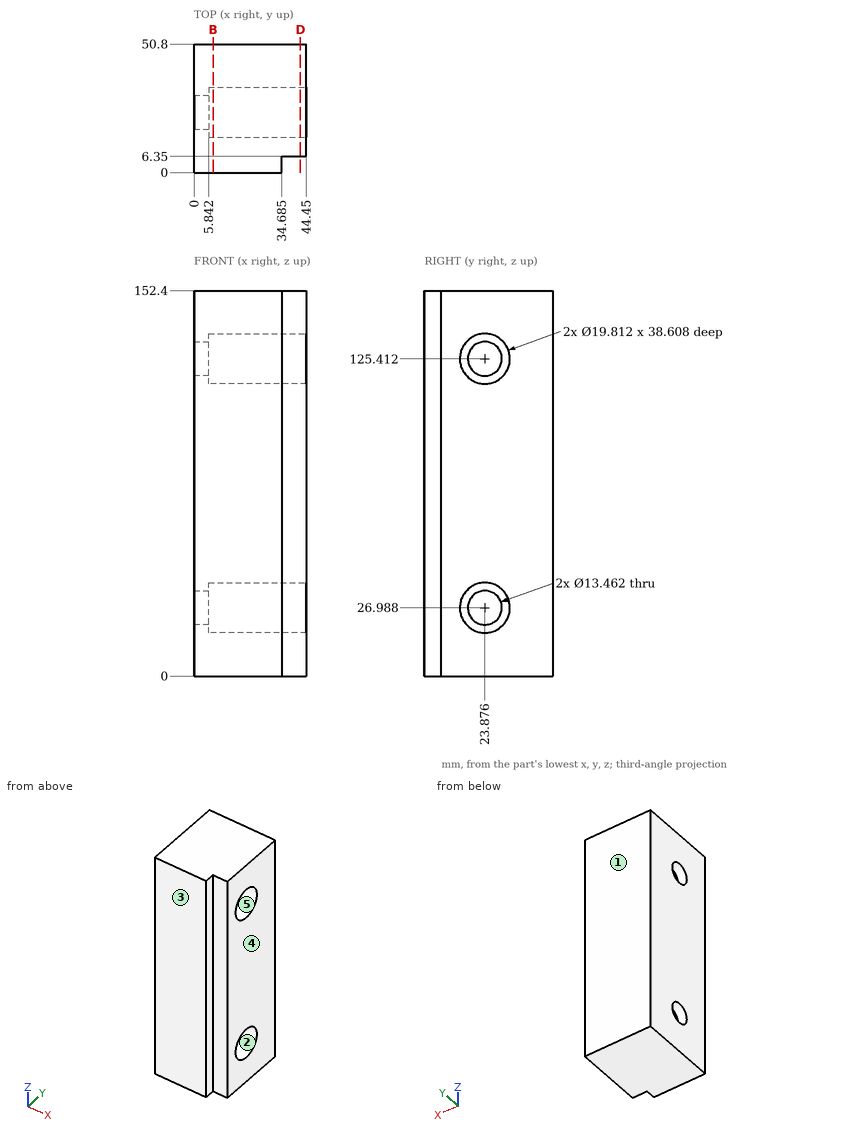
Drawing for the job (mm, zero at the part's lowest x, y, z). A direction names the side the tool comes from. Round coordinates to 2 decimals unless told otherwise and drop trailing zeros. Write each loop counter-clockwise with the first axis right and the second up, starting at its lowest first coordinate (ties: lowest second). Pieces come first, ordered by that corner, then holes. Notation, with made-up numbers: (50, 25) - (65, 25) arc R24 ccw to (65, 47) - close; hole circle Ø10 at (30, 16). An arc over 180 degrees is marked (long way). Return JSON: item names as keys, results as strings. Group by question number.
Item 1: Band-saw the part on D-D on x = 42. State how many separate pieces and enclosed holes the cut face has, plus the area to 3 significant figures.
Item 2: Flat gauge pins, fed straight in: pin 1 Ø8 at (x, z) = (40, 95.5) entering from -Y; pin 2 Ø16 at (y, z) = (24, 125) entering from +X. Where does each tip first touch, or does it go through?
Item 3: Mould opens along Y. For the marked faces 1, 2 and 3 say: +Y half, -Y half, draft (parallel to the pull), parting line (faces both ways), or undercut.
Item 4: 3-axis set-ups, long thin cutter, end or side, ignore diameter. For the marked faces 4 and 5: which of +Z, -Z, +X, -X, +Y, -Y reach the whole face in a straight line?
Item 5: Band-saw the part on B-B on x = 7.5. List the corners of the cut face in (y, z) (1 decimal).
Item 6: Probe probe 1 along Z at (x, y) = (22, 24); probe 2 along Y at (x, z) = (16.5, 125); probe 3 along Z at (x, y) = (6, 18) (1 decimal). List the from-to ranges inside material, lowest first.
Resolved:
{
 "1": {"separate pieces": "1", "enclosed holes": "2", "area": "6,160 mm²"},
 "2": {"pin 1": "stops at y = 6.35", "pin 2": "stops at x = 5.84"},
 "3": {"face 1": "+Y half", "face 2": "undercut", "face 3": "-Y half"},
 "4": {"face 4": "+Z, -Z, +X, +Y, -Y", "face 5": "+X"},
 "5": {"outline": "(0, 0) - (50.8, 0) - (50.8, 152.4) - (0, 152.4) - close; hole circle Ø19.8 at (23.9, 27); hole circle Ø19.8 at (23.9, 125.4)"},
 "6": {"probe 1": "z = 0 to 17.08, 36.89 to 115.51, 135.32 to 152.4", "probe 2": "y = 0 to 13.98, 33.77 to 50.8", "probe 3": "z = 0 to 19, 35 to 117.4, 133.4 to 152.4"}
}
